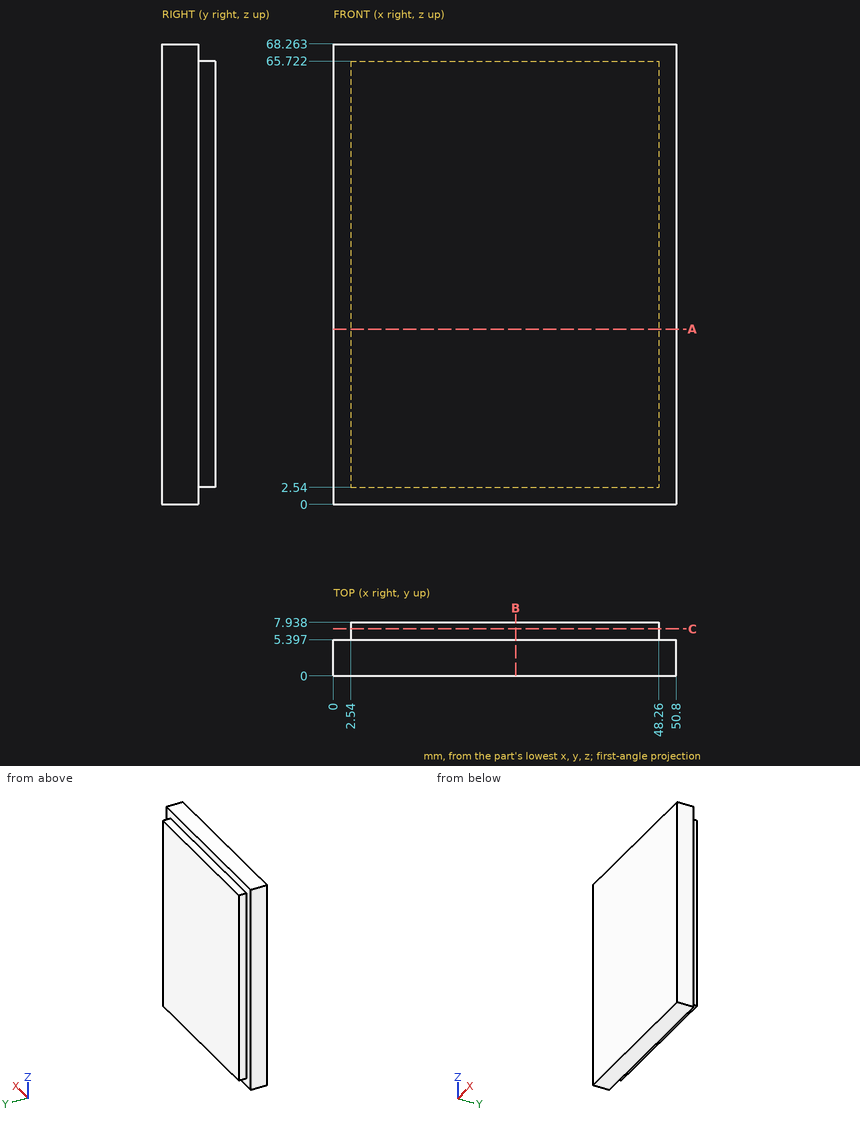
Geometry check sheet. Reference: drawing and pictorial views, mm from the part's lowest x, y, z. Coordinates: 2 decimals unless noted, no trailing zeros. Order: outer loops, then holes, each group sorted by start corner. A loop starts at its lowest first (then second) coordinate and runs counter-clockwise, first axis right, second up. Notation, with made-up numbers: (82, 0.5) - (97, 0.5) arc R18 cw to (97, 10.5) - close; hole circle Ø4 at (30, -1.75). An arc over 180 degrees is marked (long way). One line per item, written item: value.
(1) Thickness scan on probe 1 along X at (y, z) = (6.75, 39.5); probe 2 along Z at (x, y) = (33, 5.75). Record the ranges inside material, lowest first. Write a range as from..to.
Data:
probe 1: x = 2.54..48.26
probe 2: z = 2.54..65.72
(2) Sectioned sample at B-B (x = 27). Enter the section's corners in (y, z).
Data:
outline: (0, 0) - (5.4, 0) - (5.4, 2.54) - (7.94, 2.54) - (7.94, 65.72) - (5.4, 65.72) - (5.4, 68.26) - (0, 68.26) - close
(3) Sectioned sample at A-A (z = 26). Enter the section's corners in (x, y).
Data:
outline: (0, 0) - (50.8, 0) - (50.8, 5.4) - (48.26, 5.4) - (48.26, 7.94) - (2.54, 7.94) - (2.54, 5.4) - (0, 5.4) - close
(4) Sectioned sample at C-C (y = 7). Enter the section's corners in (x, z).
Data:
outline: (2.54, 2.54) - (48.26, 2.54) - (48.26, 65.72) - (2.54, 65.72) - close
(5) Depth check by flat-ended pin: pin 1 Ø1.3 at (y, z) = (7, 26) entering from +X; pin 2 Ø1.3 at (y, z) = (7, 30) entering from -X; pin 3 Ø1.3 at (x, y) = (30.5, 7) entering from +Z. Enter the tip coordinate at first touch or a pass-through.
Data:
pin 1: stops at x = 48.26
pin 2: stops at x = 2.54
pin 3: stops at z = 65.72
